from build123d import *

# Parameters (mm, degrees)
F1_DEPTH      = 50.8
F1_DEPTH_BACK = 50.8


with BuildPart() as f1:
    # F0 (on Front) → F1 (new body, two sides)
    with BuildSketch(Plane.XZ) as f1_sk:
        Polygon((-101.6, 50.8), (-101.6, 0), (101.6, 0), (101.6, 50.8), (76.2, 50.8), (76.2, 25.4), (-76.2, 25.4), (-76.2, 50.8), align=None)
    extrude(amount=F1_DEPTH)
    extrude(f1_sk.sketch, amount=-F1_DEPTH_BACK)


solid = f1.part
The listing builds one solid part. Answer for the finished solid, in the listing's coordinates (mm). A direction names the side the tool comes from. Give positions to 0.01 mm unless a question says otherwise; leave off trailing zeros. Write each loop counter-clockwise with the first axis right and the second up, starting at its lowest first coordinate (ties: lowest second). Pieces come first, ordered by that corner, then holes.
Item 1: Which of the six approach directions +Z, -Z, +X, -X, +Y, -Y give full straight-line access (tool end or side, diameter ignored) to faces 1 (the flat face through (-1, -1, 0)), 2 (the flat face through (-76.2, -1, 38))?
Item 2: Find the intervals of material crossed by line 1 along X through (y, z) = (-33, 26); line 2 along Z through (x, y) = (-14, 32), in increasing order.
Item 3: A flat-ended cylindrical pin translates along its axis: P1, Ø1, axis at x = 67, y = 19.5, coming from the +Z side. Find the tip coordinate at first contact, or state that the pin passes through.
Item 4: Determine the mould class of faces 3 (the flat face through (76.2, -1, 38)), 4 (the flat face through (-1, -50.8, 14)), 5 (the flat face through (-101.6, -1, 26)) for opening direction X: released by +X, released by -X, zero draft, split by the parting line, or undercut.
Item 5: Section A-A, the plane z = 47 is taken. Write down the section's boundary in (x, y).
Item 6: Section C-C, the plane x = 61 is taken. Write down the section's boundary in (y, z).
Item 7: Section B-B, the plane y = -11 is taken. Write down the section's boundary in (x, z).
Completed:
1. face 1: -Z, +X, -X, +Y, -Y
1. face 2: +Z, +Y, -Y
2. line 1: x = -101.6 to -76.2, 76.2 to 101.6
2. line 2: z = 0 to 25.4
3. P1: stops at z = 25.4
4. face 3: undercut
4. face 4: zero draft
4. face 5: released by -X
5. outline: (-101.6, -50.8) - (-76.2, -50.8) - (-76.2, 50.8) - (-101.6, 50.8) - close; (76.2, -50.8) - (101.6, -50.8) - (101.6, 50.8) - (76.2, 50.8) - close
6. outline: (-50.8, 0) - (50.8, 0) - (50.8, 25.4) - (-50.8, 25.4) - close
7. outline: (-101.6, 0) - (101.6, 0) - (101.6, 50.8) - (76.2, 50.8) - (76.2, 25.4) - (-76.2, 25.4) - (-76.2, 50.8) - (-101.6, 50.8) - close
